from build123d import *

# Parameters (mm, degrees)
PAD_DEPTH = 2.5


with BuildPart() as part:
    # Sketch → Pad (new body, symmetric)
    with BuildSketch(Plane.XY):
        with BuildLine():
            Line((91.25, 76.5), (-91.25, 76.5))
            Line((-91.25, 76.5), (-91.25, 71.5))
            Line((-91.25, 71.5), (-121.25, 71.5))
            Line((-121.25, 71.5), (-121.25, 46.5))
            Line((-121.25, 46.5), (-126.25, 46.5))
            Line((-126.25, 46.5), (-126.25, -46.5))
            Line((-126.25, -46.5), (-121.25, -46.5))
            Line((-121.25, -46.5), (-121.25, -71.5))
            Line((-121.25, -71.5), (-91.25, -71.5))
            Line((-91.25, -71.5), (-91.25, -76.5))
            Line((-91.25, -76.5), (91.25, -76.5))
            Line((91.25, -76.5), (91.25, -71.5))
            Line((91.25, -71.5), (121.25, -71.5))
            Line((121.25, -71.5), (121.25, -6))
            Line((100.75, -6), (121.25, -6))
            ThreePointArc((100.75, 32), (81.75, 13), (100.75, -6))
            Line((121.25, 32), (100.75, 32))
            Line((121.25, 32), (121.25, 71.5))
            Line((121.25, 71.5), (91.25, 71.5))
            Line((91.25, 71.5), (91.25, 76.5))
        make_face()
    extrude(amount=PAD_DEPTH, both=True)


solid = part.part
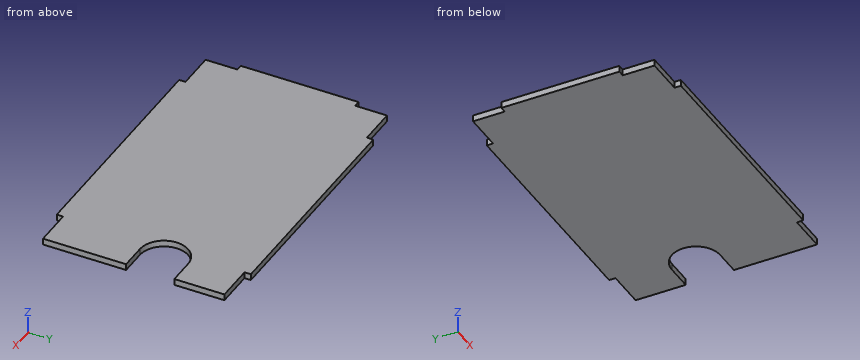
Read the model definition and answer for the solid it produces. Units are mm, in the model's axes. Round coordinates to 2 decimals unless told otherwise and drop trailing zeros. Loops run counter-clockwise (first coordinate to the right, second up) from the corner with the lowest first, then second, coordinate; pieces in that order, holes last.
Q1. Section B-B on x = -94 is taken. Write down the section's boundary in (y, z), and give its area (3 significant figures).
Q2. Section C-C on y = 13 is taken. Write down the section's boundary in (x, z), and give its area (3 significant figures).
Q3. Section A-A on z = -0.2 is taken. Write down the section's boundary in (x, y), and give its area (3 significant figures).
Q4. Consider probe 1 along Y at (x, z) = (106.5, 1.15); probe 2 along X at (y, z) = (-54.5, -1.85); probe 3 along X at (y, z) = (0, -1.9). Determine where each line is inside the solid, lowest interval first.
Q5. Each of these flat-tipped pins is pushed along its axis until it touches: pin 1 (1.5 mm diameter, centred on y = -62, z = -1, fed in from -X); pin 2 (1.5 mm diameter, centred on y = -75, z = -0.5, fed in from +X); pin 3 (2.5 mm diameter, centred on x = -107.5, z = -0.5, fed in from +Y). Where does it stop, or does it pass through?
Output:
1. outline: (-71.5, -2.5) - (71.5, -2.5) - (71.5, 2.5) - (-71.5, 2.5) - close
1. area: 715 mm2
2. outline: (-126.25, -2.5) - (81.75, -2.5) - (81.75, 2.5) - (-126.25, 2.5) - close
2. area: 1,040 mm2
3. outline: (-126.25, -46.5) - (-121.25, -46.5) - (-121.25, -71.5) - (-91.25, -71.5) - (-91.25, -76.5) - (91.25, -76.5) - (91.25, -71.5) - (121.25, -71.5) - (121.25, -6) - (100.75, -6) arc R19 cw to (100.75, 32) - (121.25, 32) - (121.25, 71.5) - (91.25, 71.5) - (91.25, 76.5) - (-91.25, 76.5) - (-91.25, 71.5) - (-121.25, 71.5) - (-121.25, 46.5) - (-126.25, 46.5) - close
3. area: 35,600 mm2
4. probe 1: y = -71.5 to -6, 32 to 71.5
4. probe 2: x = -121.25 to 121.25
4. probe 3: x = -126.25 to 86.89
5. pin 1: stops at x = -121.25
5. pin 2: stops at x = 91.25
5. pin 3: stops at y = 71.5
